Here's how the part is built. I have some questions about the finished solid (model axes, mm). Face numbers are marked on the shaded views. A direction names the side the tool comes from. Round coordinates to 2 decimals unless told otherwise and drop trailing zeros. Loops run counter-clockwise (first coordinate to the right, second up) from the corner with the lowest first, then second, coordinate; pieces in that order, holes last. Notation, with made-up numbers: M 14.5,69 L 30.5,69 A22 cw 30.5,108 Z; hole C -31,44 d3. An arc over 180 degrees is marked long. Use a Markdown table: item, result.
```python
from build123d import *

# Parameters (mm, degrees)
F1_DEPTH = 6
F2_R     = 4
F3_DEPTH = 6.001
F4_R     = 8
F5_DEPTH = 45


# Not quite as in the source:
# - a feature names something its author has since deleted; it is built from what else it names


with BuildPart() as f1:
    # F0 (on Top) → F1 (new body)
    with BuildSketch(Plane.XY):
        Polygon((-19, 56), (-19, 0), (-19, -56), (0, -56), (19, -56), (19, 0), (19, 56), (0, 56), align=None)
    extrude(amount=F1_DEPTH)

    # F2 (on face) → F3 (cut, through all)
    with BuildSketch(Plane.XY.offset(6)):
        with Locations((0, 38.5)):
            Circle(F2_R)
        with Locations((0, -38.5)):
            Circle(F2_R)
    extrude(amount=-F3_DEPTH, mode=Mode.SUBTRACT)

    # F4 (on face) → F5 (join)
    with BuildSketch(Plane.XY.offset(6)):
        with Locations((0, 18)):
            Circle(F4_R)
    extrude(amount=F5_DEPTH)


solid = f1.part
```
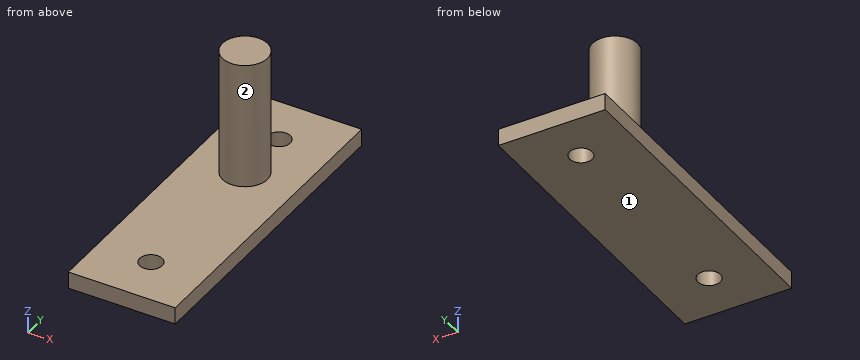
Q1. For the marked faces 1 and 2, which set-ups out of +Z, -Z, +X, -X, +Y, -Y let a thin tool reach every point of the face, with its end or its side?
Return value:
| item | result |
|---|---|
| face 1 | -Z, +X, -X, +Y, -Y |
| face 2 | +Z |
Q2. Imagine slicing it at B-B, the plane x = 0. Please give me the cut outline in (y, z).
Return value:
| item | result |
|---|---|
| outline | M -56,0 L -42.5,0 L -42.5,6 L -56,6 Z; M -34.5,0 L 34.5,0 L 34.5,6 L 26,6 L 26,51 L 10,51 L 10,6 L -34.5,6 Z; M 42.5,0 L 56,0 L 56,6 L 42.5,6 Z |
Q3. Imagine slicing it at D-D, the plane x = -14.5. Please give me the cut outline in (y, z).
Return value:
| item | result |
|---|---|
| outline | M -56,0 L 56,0 L 56,6 L -56,6 Z |
Q4. Imagine slicing it at A-A, the plane y = 38.5. Please give me the cut outline in (x, z), then the cut area to 3 significant figures.
Return value:
| item | result |
|---|---|
| outline | M -19,0 L -4,0 L -4,6 L -19,6 Z; M 4,0 L 19,0 L 19,6 L 4,6 Z |
| area | 180 mm^2 |
Q5. Will these pins go through, and if not, where does the flat tip stop? P1, Ø13, axis at x = 0, y = 38.5, coming from the +Z side; P2, Ø8, axis at x = -12.5, z = 33.5, coming from the -Y side; P3, Ø8, axis at x = -11, z = 22.5, coming from the +Y side.
Return value:
| item | result |
|---|---|
| P1 | stops at z = 6 |
| P2 | passes through |
| P3 | stops at y = 21.87 |
Q6. I need wall thicknesses on line 1 (Y direction, x = 0, z = 3); line 2 (Z direction, x = -17, y = 29); line 3 (X direction, y = 38, z = 3). Which ranges of each line are inside material? Lowest first, please. Write a range as from..to.
Return value:
| item | result |
|---|---|
| line 1 | y = -56..-42.5, -34.5..34.5, 42.5..56 |
| line 2 | z = 0..6 |
| line 3 | x = -19..-3.97, 3.97..19 |
Q7. Imagine slicing it at C-C, the plane z = 41.5. Please give me the cut outline in (x, y), then the cut area to 3 significant figures.
Return value:
| item | result |
|---|---|
| outline | C 0,18 d16 |
| area | 201 mm^2 |
